from build123d import *

# Parameters (mm, degrees)
SKETCH1_W           = 21
SKETCH1_H           = 14
BOSS_EXTRUDE1_DEPTH = 50
SKETCH2_R           = 1.75
CUT_EXTRUDE1_DEPTH  = 100
SKETCH3_R           = 1.75
CUT_EXTRUDE2_DEPTH  = 22


with BuildPart() as part:
    # Sketch1 → Boss-Extrude1 (new body)
    with BuildSketch(Plane(origin=(0, 0, 0), x_dir=(1, 0, 0), z_dir=(0, 1, 0))):
        with Locations((-0.5, 4.045454545)):
            Rectangle(SKETCH1_W, SKETCH1_H)
    extrude(amount=BOSS_EXTRUDE1_DEPTH)

    # Sketch2 → Cut-Extrude1 (cut)
    with BuildSketch(Plane.XY.offset(2.954545455)):
        with Locations((0, 2.5)):
            Circle(SKETCH2_R)
        with Locations((0, 20)):
            Circle(SKETCH2_R)
    extrude(amount=-CUT_EXTRUDE1_DEPTH, mode=Mode.SUBTRACT)

    # Sketch3 → Cut-Extrude2 (cut)
    with BuildSketch(Plane(origin=(0, 0, -11.045454545), x_dir=(-1, 0, 0), z_dir=(0, 0, -1))):
        with Locations((0, 43.5)):
            Circle(SKETCH3_R)
    extrude(amount=-CUT_EXTRUDE2_DEPTH, mode=Mode.SUBTRACT)


solid = part.part
Verification items for the finished model (mm, model axes). Coordinates: 2 decimals unless noted, no trailing zeros. Order: outer loops, then holes, each group sorted by start corner. A loop starts at its lowest first (then second) coordinate and runs counter-clockwise, first axis right, second up. Notation, with made-up numbers: (-32.5, 34.5) -> (-7.5, 34.5) arc R27 ccw to (-7.5, 63.5) -> close; hole circle Ø2 at (-28.5, 22.5). An arc over 180 degrees is marked (long way). Put each result on its own line as item: value. Start each with the question number.
1. Mould release check, pull along X, two halves, no side actions. Record for faces 1 (the cylindrical face through (0.81, 0.95, -3.95)), 2 (the flat face through (-1, 25, 2.955)), 3 (the flat face through (-11, 25, -4)): released by +X, released by -X, zero draft, split by the parting line, or undercut.
2. Go/stop test with a flat-tipped pin: pin 1 Ø6 at (x, z) = (-3.5, -1.5) entering from -Y. Record where the tip stops, or that it passes through.
3. Cross-section at B-B, the plane y = 43.5. Record the boundary of the cut face in (x, z).
4. Material ranges on L1, parallel to Y at x = 0, z = -2; L2, parallel to Y at x = -1, z = -10.25; L3, parallel to X at y = 19, z = -5, recorded low to high. Write a range as [from, to].
5. Cross-section at A-A, the plane z = -0.25. Record the boundary of the cut face in (x, y).
6. Cross-section at C-C, the plane x = 0. Record the boundary of the cut face in (y, z), then the cut area to 3 significant figures.
Computed:
1. face 1: undercut
1. face 2: zero draft
1. face 3: released by -X
2. pin 1: y = 0
3. outline: (-11, -11.05) -> (-1.75, -11.05) -> (-1.75, 2.95) -> (-11, 2.95) -> close; (1.75, -11.05) -> (10, -11.05) -> (10, 2.95) -> (1.75, 2.95) -> close
4. L1: [0, 0.75], [4.25, 18.25], [21.75, 41.75], [45.25, 50]
4. L2: [0, 1.06], [3.94, 18.56], [21.44, 42.06], [44.94, 50]
4. L3: [-11, -1.44], [1.44, 10]
5. outline: (-11, 0) -> (10, 0) -> (10, 50) -> (-11, 50) -> close; hole circle Ø3.5 at (0, 2.5); hole circle Ø3.5 at (0, 20); hole circle Ø3.5 at (0, 43.5)
6. outline: (0, -11.05) -> (0.75, -11.05) -> (0.75, 2.95) -> (0, 2.95) -> close; (4.25, -11.05) -> (18.25, -11.05) -> (18.25, 2.95) -> (4.25, 2.95) -> close; (21.75, -11.05) -> (41.75, -11.05) -> (41.75, 2.95) -> (21.75, 2.95) -> close; (45.25, -11.05) -> (50, -11.05) -> (50, 2.95) -> (45.25, 2.95) -> close
6. area: 553 mm2
